from build123d import *

# Parameters (mm, degrees)
F1_DEPTH = 4.7625
F2_W     = 19.05
F2_H     = 6.35
F3_DEPTH = 25.4
F4_R     = 2.54
F9_R     = 1.26999


# Not quite as in the source:
# - a fillet or chamfer is up to 0.001 mm smaller than in the source, because OpenCascade refuses the exact size


with BuildPart() as f1:
    # F0 (on Top) → F1 (new body, symmetric)
    with BuildSketch(Plane.XY):
        with BuildLine():
            Line((101.6, 0), (0, 0))
            Line((0, 0), (0, -50.8))
            Line((0, -50.8), (50.8, -50.8))
            ThreePointArc((50.8, -50.8), (86.7210244843, -35.9210244843), (101.6, 0))
        make_face()
    extrude(amount=F1_DEPTH, both=True)

    # F2 (on face) → F3 (cut)
    with BuildSketch(Plane(origin=(0, 0, 0), x_dir=(0, -1, 0), z_dir=(-1, 0, 0))):
        with Locations((12.7, 0)):
            Rectangle(F2_W, F2_H)
    extrude(amount=-F3_DEPTH, mode=Mode.SUBTRACT)

    # F4
    f4_edges = [f1.edges().sort_by_distance(p)[0] for p in [
        (12.7, -3.175, 3.175),
        (12.7, -22.225, 3.175),
        (12.7, -3.175, -3.175),
        (12.7, -22.225, -3.175),
    ]]
    fillet(f4_edges, radius=F4_R)


with BuildPart() as f6:
    # F6: sweep along a path in F6_path
    with BuildLine(Plane(origin=(50.8, -50.8, 4.7625), x_dir=(0, 1, 0), z_dir=(0, 0, 1))) as f6_path:
        Line((0, 50.8), (0, 0))
        ThreePointArc((0, 0), (14.8789755157, -35.9210244843), (50.8, -50.8))
    # F5 (on face) → F6 (sweep)
    with BuildSketch(Plane(origin=(0, 0, 0), x_dir=(0, -1, 0), z_dir=(-1, 0, 0))):
        with BuildLine():
            Line((50.8, 4.7625), (25.4, 4.7625))
            ThreePointArc((25.4, 4.7625), (37.9805074569, 2.1472133229), (50.8, 1.27))
            Line((50.8, 1.27), (50.8, 4.7625))
        make_face()
    sweep(path=f6_path.line)


with BuildPart() as f7_1:
    # F7: instance of F6
    add(f6.part.mirror(Plane.XY))


with BuildPart() as f1_1:
    add(f1.part)

    # F8: cut F6, F7_1
    add(f6.part, mode=Mode.SUBTRACT)
    add(f7_1.part, mode=Mode.SUBTRACT)

    # F9 (radius 1.27 in the source; OpenCascade refuses exactly that, so slightly less here)
    f9_edges = [f1_1.edges().sort_by_distance(p)[0] for p in [
        (38.1, 0, 4.7625),
        (38.1, 0, -4.7625),
        (88.780507, 0, 2.147213),
        (88.780507, 0, -2.147213),
        (25.4, -50.8, 1.27),
        (25.4, -50.8, -1.27),
        (86.721024, -35.921024, 1.27),
        (86.721024, -35.921024, -1.27),
    ]]
    fillet(f9_edges, radius=F9_R)


solid = f1_1.part
Work out the finished part from the listing and answer in its coordinate system (mm). A direction names the side the tool comes from. Coordinates: 2 decimals unless noted, no trailing zeros. Use one line per item in the form item = value. Start each with the question number.
1. Each of these flat-tipped pins is pushed along its axis until it touches: P1, Ø1.5, axis at y = -22.5, z = 1, coming from the +X side; P2, Ø4, axis at y = -33.5, z = 2, coming from the +X side; P3, Ø1, axis at x = 22.5, y = -34.5, coming from the +Z side. Where does it stop, or does it pass through?
2. Straight lines are drawn through the part: probe 1 along Z at (x, y) = (11, -9) (1 decimal); probe 2 along X at (y, z) = (-20, -0.25); probe 3 along X at (y, z) = (-45, 0.5). For each, find the intervals that lie inside material, in ascending order. Write a range as from..to.
3. The mould has two halves that part along Z. Classify faces 1 (the face through (25.4, -13, 0)), 2 (the face through (38, -13, -4.762)), 3 (the face through (25.76, -37.53, 2.21)): released by +Z, released by -Z, zero draft, split by the parting line, or undercut.
4. A tool of negligible diameter and unlimited length cuts with its end or side. For faces 4 (the face through (12.88, -3.94, 2.45)), 5 (the face through (38, -13, 4.762)), from which of +Z, -Z, +X, -X, +Y, -Y can it reach the whole face along a straight path? Write none if from no direction.
Evaluation:
q1.P1 = 96.51
q1.P2 = 90.01
q1.P3 = 2.78
q2.probe_1 = -4.8..-3.2, 3.2..4.8
q2.probe_2 = 25.4..97.47
q2.probe_3 = 0..74.16
q3.face_1 = undercut
q3.face_2 = released by -Z
q3.face_3 = released by +Z
q4.face_4 = -X
q4.face_5 = +Z, +X, -X, +Y, -Y
